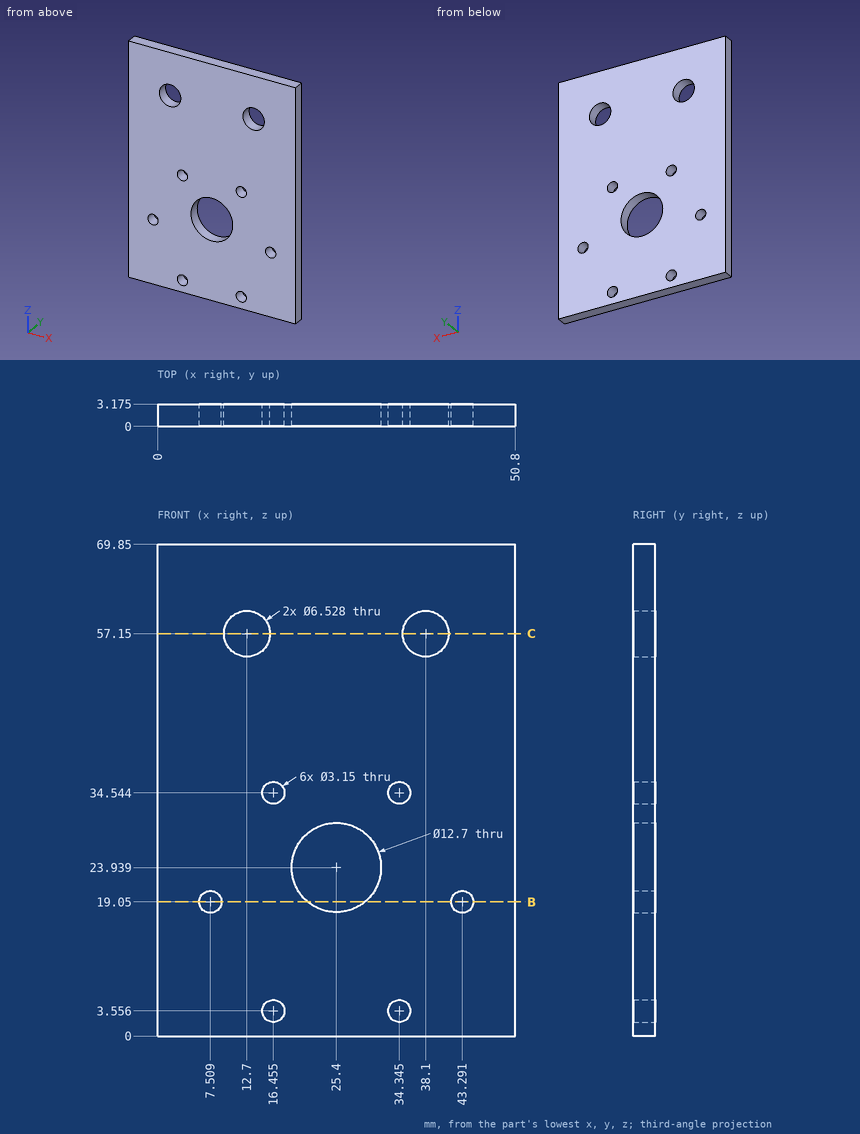
The drawing under review shows one solid part. Ordinate dimensions are in mm from its lowest x, y, z. Give positions to 0.01 mm unless a question says otherwise; leave off trailing zeros. Write each loop counter-clockwise with the first axis right and the second up, starting at its lowest first coordinate (ties: lowest second). Pieces come first, ordered by that corner, then holes.
1. Add section C-C, the plane z = 57.15. Write out the cut boundary in (x, y) (1 decimal), plus the area to 3 significant figures.
2. Wall thickness on L1, parallel to Z at x = 38.1, y = 2.55; L2, parallel to X at y = 2.35, z = 57; L3, parallel to Z at x = 25.4, y = 1.4: over which ranges is each line inside the solid? List them lowest first.
3. Add section B-B, the plane z = 19.05. Write out the cut boundary in (x, y) (1 decimal).
Worked answers:
1. outline: (0, 0) - (9.4, 0) - (9.4, 3.2) - (0, 3.2) - close; (16, 0) - (34.8, 0) - (34.8, 3.2) - (16, 3.2) - close; (41.4, 0) - (50.8, 0) - (50.8, 3.2) - (41.4, 3.2) - close
1. area: 120 mm2
2. L1: z = 0 to 53.89, 60.41 to 69.85
2. L2: x = 0 to 9.44, 15.96 to 34.84, 41.36 to 50.8
2. L3: z = 0 to 17.59, 30.29 to 69.85
3. outline: (0, 0) - (5.9, 0) - (5.9, 3.2) - (0, 3.2) - close; (9.1, 0) - (21.3, 0) - (21.3, 3.2) - (9.1, 3.2) - close; (29.5, 0) - (41.7, 0) - (41.7, 3.2) - (29.5, 3.2) - close; (44.9, 0) - (50.8, 0) - (50.8, 3.2) - (44.9, 3.2) - close
